Check sheet for the drawn part. Datum: minimum x, y, z corner. Units: mm. Coordinates: 2 decimals unless noted, no trailing zeros. Loops run counter-clockwise (first coordinate to the right, second up) from the corner with the lowest first, then second, coordinate; pieces in that order, holes last. Notation, with made-up numbers: (42, 63.25) -> (63, 63.25) arc R20 ccw to (63, 85.25) -> close; hole circle Ø5 at (84, -22). An arc over 180 degrees is marked (long way). Use CSV: the item, a comma, the result in double quotes. Start each with the question number.
1. Thickness scan on L1, parallel to X at y = 5, z = 3.5; L2, parallel to X at y = 5.5, z = 34; L3, parallel to Z at x = 10, y = 2.95. Record the ranges inside material, lowest first.
2. Sectioned sample at C-C, the plane y = 8. Record the cut outline in (x, z).
3. Sectioned sample at A-A, the plane x = 10. Record the cut outline in (y, z).
4. Sectioned sample at B-B, the plane z = 21.5. Record the cut outline in (x, y).
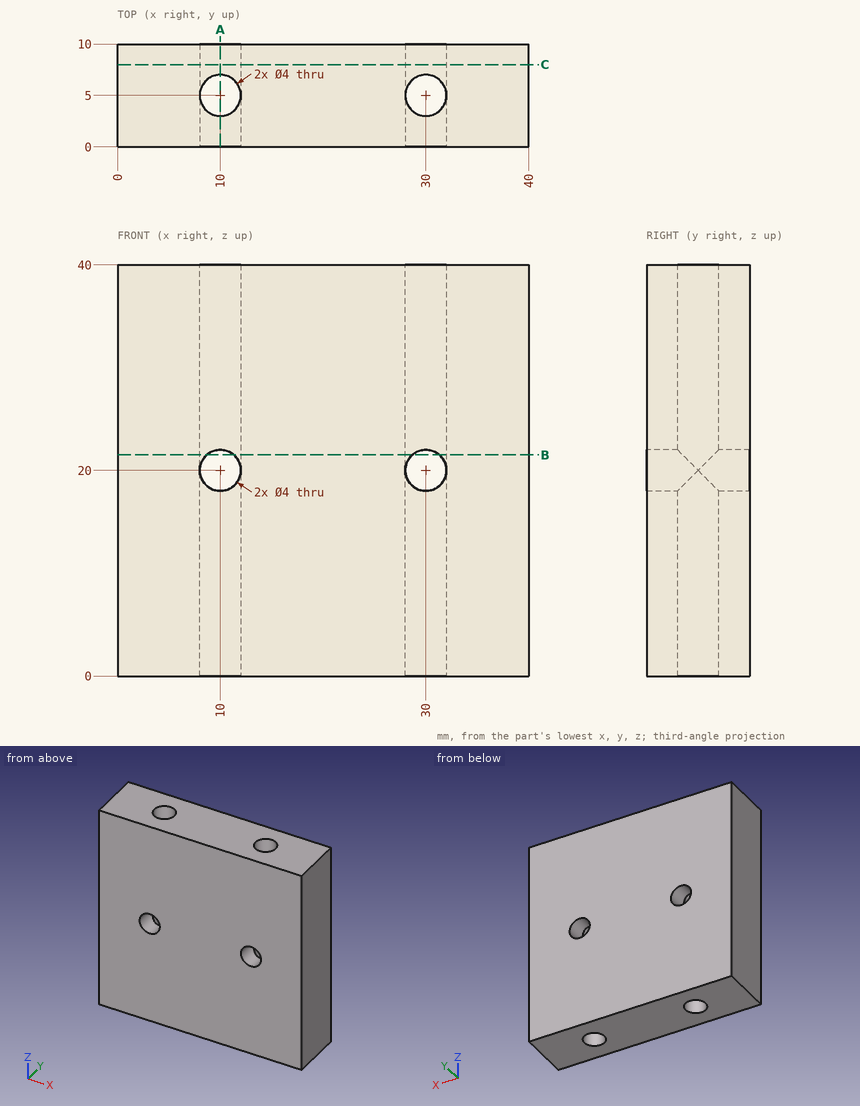
Completed:
1,L1,"0 to 8, 12 to 28, 32 to 40"
1,L2,"0 to 8.06, 11.94 to 28.06, 31.94 to 40"
1,L3,"0 to 18, 22 to 40"
2,outline,"(0, 0) -> (40, 0) -> (40, 40) -> (0, 40) -> close; hole circle Ø4 at (10, 20); hole circle Ø4 at (30, 20)"
3,outline,"(0, 0) -> (3, 0) -> (3, 18) -> (0, 18) -> close; (0, 22) -> (3, 22) -> (3, 40) -> (0, 40) -> close; (7, 0) -> (10, 0) -> (10, 18) -> (7, 18) -> close; (7, 22) -> (10, 22) -> (10, 40) -> (7, 40) -> close"
4,outline,"(0, 0) -> (8.68, 0) -> (8.68, 3.5) arc R2 cw to (8.68, 6.5) -> (8.68, 10) -> (0, 10) -> close; (11.32, 0) -> (28.68, 0) -> (28.68, 3.5) arc R2 cw to (28.68, 6.5) -> (28.68, 10) -> (11.32, 10) -> (11.32, 6.5) arc R2 cw to (11.32, 3.5) -> close; (31.32, 0) -> (40, 0) -> (40, 10) -> (31.32, 10) -> (31.32, 6.5) arc R2 cw to (31.32, 3.5) -> close"
